Check sheet for the modelled part. Datum: model origin and axes. Units: mm. A direction names the side the tool comes from. Round coordinates to 2 decimals unless told otherwise and drop trailing zeros. Loops run counter-clockwise (first coordinate to the right, second up) from the corner with the lowest first, then second, coordinate; pieces in that order, holes last. Notation, with made-up numbers: (17.25, -13) -> (45.25, -13) arc R12 ccw to (45.25, 2) -> close; hole circle Ø7 at (-2.75, -35.5). An arc over 180 degrees is marked (long way). Return JSON: item names as keys, results as strings.
Autodesk Inventor part; units mm, degrees
ref_plane "YZ Plane" through (0, 0, 0) normal (1, 0, 0) x (0, 1, 0)
ref_plane "XZ Plane" through (0, 0, 0) normal (0, 1, 0) x (-1, 0, 0)
ref_plane "XY Plane" through (0, 0, 0) normal (0, 0, 1) x (1, 0, 0)
sketch "Sketch1" plane through (0, 0, 0) normal (1, 0, 0) x (0, 1, 0)
  line L0 (920.75, 0) -> (0, 0)
  line L1 (0, 0) -> (920.75, 0)
  line L2 (-297.6389, 409.8513) -> (2710.7909, 409.8513) construction
  line L3 (2710.7909, 409.8513) -> (2710.7909, -1716.9746) construction
  line L4 (2710.7909, -1716.9746) -> (-297.6389, -1716.9746) construction
  line L5 (-297.6389, -1716.9746) -> (-297.6389, 409.8513) construction
  line L6 (0, 0) -> (920.75, 0)
  line L7 (920.75, 0) -> (920.75, 100.33)
  line L8 (0, 100.33) -> (920.75, 100.33)
  line L9 (0, 0) -> (0, 100.33)
  line L10 (0, 100.33) -> (0, 120.65)
  line L11 (0, 120.65) -> (920.75, 120.65)
  line L12 (920.75, 120.65) -> (920.75, 100.33)
  line L13 (0, 120.65) -> (0, 196.85)
  line L14 (920.75, 196.85) -> (920.75, 120.65)
  line L15 (477.9962, 0) -> (477.9962, -13.97)
  line L16 (477.9962, -13.97) -> (434.8162, -13.97)
  line L17 (434.8162, -13.97) -> (434.8162, 0)
  line L18 (133.294, 0) -> (133.294, -13.97)
  line L19 (133.294, -13.97) -> (90.114, -13.97)
  line L20 (90.114, -13.97) -> (90.114, 0)
  line L21 (769.0257, 0) -> (769.0257, -13.97)
  line L22 (769.0257, -13.97) -> (812.2057, -13.97)
  line L23 (812.2057, -13.97) -> (812.2057, 0)
  line L24 (434.8162, -13.97) -> (477.9962, -13.97)
  line L25 (769.0257, -13.97) -> (812.2057, -13.97)
  line L26 (90.114, -13.97) -> (133.294, -13.97)
  line L27 (90.114, -13.97) -> (111.704, -13.97)
  line L28 (111.704, -13.97) -> (100.909, -13.97)
  line L29 (100.909, -13.97) -> (122.499, -13.97)
  line L30 (122.499, -13.97) -> (122.499, -33.02)
  line L31 (122.499, -33.02) -> (100.909, -33.02)
  line L32 (100.909, -33.02) -> (100.909, -13.97)
  line L33 (434.8162, -13.97) -> (456.4062, -13.97)
  line L34 (456.4062, -13.97) -> (445.6112, -13.97)
  line L35 (445.6112, -13.97) -> (467.2012, -13.97)
  line L36 (467.2012, -13.97) -> (467.2012, -33.02)
  line L37 (467.2012, -33.02) -> (445.6112, -33.02)
  line L38 (445.6112, -33.02) -> (445.6112, -13.97)
  line L39 (769.0257, -13.97) -> (790.6157, -13.97)
  line L40 (790.6157, -13.97) -> (779.8207, -13.97)
  line L41 (779.8207, -13.97) -> (801.4107, -13.97)
  line L42 (801.4107, -13.97) -> (801.4107, -33.02)
  line L43 (801.4107, -33.02) -> (779.8207, -33.02)
  line L44 (779.8207, -33.02) -> (779.8207, -13.97)
  line L45 (434.8162, 0) -> (413.2262, 0)
  line L46 (413.2262, 0) -> (413.2262, -11.43)
  line L47 (413.2262, -11.43) -> (371.9512, -11.43)
  line L48 (371.9512, -11.43) -> (371.9512, 64.77)
  arc A0 (413.2262, 72.0379) -> (371.9512, 72.0379) centre (392.5887, 68.404) ccw
  line L49 (413.2262, 0) -> (413.2262, 64.77)
  line L50 (371.9512, 64.77) -> (371.9512, 72.0379)
  line L51 (413.2262, 64.77) -> (413.2262, 72.0379)
  line L52 (434.8162, -13.97) -> (434.8162, 202.565)
  line L53 (477.9962, -13.97) -> (477.9962, 202.565)
  line L54 (769.0257, -13.97) -> (769.0257, 202.565)
  line L55 (812.2057, -13.97) -> (812.2057, 202.565)
  line L56 (812.2057, 202.565) -> (769.0257, 202.565)
  line L57 (477.9962, 202.565) -> (434.8162, 202.565)
  line L58 (133.294, -13.97) -> (133.294, 182.245)
  line L59 (90.114, -13.97) -> (90.114, 182.245)
  line L60 (90.114, 182.245) -> (133.294, 182.245)
  line L61 (67.3834, 182.245) -> (164.6776, 182.245)
  line L62 (413.2262, 202.565) -> (508.4774, 202.565)
  line L63 (745.5808, 202.565) -> (847.3717, 202.565)
  line L64 (67.3834, 161.925) -> (164.6776, 161.925)
  line L65 (413.2262, 182.245) -> (508.4774, 182.245)
  line L66 (745.5808, 182.245) -> (847.3717, 182.245)
  line L67 (133.294, -13.97) -> (133.294, 78.74)
  line L68 (133.294, 78.74) -> (434.8162, 78.74)
  line L69 (133.294, -13.97) -> (133.294, 26.67)
  line L70 (133.294, 26.67) -> (371.9512, 26.67)
  line L71 (133.294, 26.67) -> (298.394, 26.67)
  line L72 (298.394, 26.67) -> (317.7759, 78.74)
  line L73 (133.294, 78.74) -> (133.294, 59.055)
  line L74 (133.294, 59.055) -> (310.4486, 59.055)
  line L75 (371.9512, 0) -> (371.9512, -5.715)
  line L76 (371.9512, -5.715) -> (413.2262, -5.715)
  dimension "d0" = 920.75
  dimension "d1" = 20.32
  dimension "d2" = 76.2
  dimension "d3" = 13.97
  dimension "d4" = 43.18
  dimension "d5" = 13.97
  dimension "d6" = 43.18
  dimension "d7" = 13.97
  dimension "d8" = 13.97
  dimension "d9" = 43.18
  dimension "d10" = 21.59
  dimension "d11" = 19.05
  dimension "d12" = 21.59
  dimension "d13" = 19.05
  dimension "d14" = 21.59
  dimension "d15" = 19.05
  dimension "d16" = 21.59
  dimension "d17" = 11.43
  dimension "d18" = 41.275
  dimension "d19" = 76.2
  dimension "d20" = 20.955
  dimension "d21" = 216.535
  dimension "d22" = 216.535
  dimension "d23" = 216.535
  dimension "d24" = 216.535
  dimension "d25" = 196.215
  dimension "d26" = 20.32
  dimension "d27" = 20.32
  dimension "d28" = 20.32
  dimension "d29" = 92.71
  dimension "d30" = 40.64
  dimension "d31" = 165.1
  dimension "d32" = 19.685
extrude "Extrusion1" add sketch "Sketch1" along normal blind 5.715 and the other way blind 145.415 contours L46 L76 L48 L0 | L0 L48 L50 A0 L68 L51 L49 | L68 A0
sketch "Sketch2" plane through (-145.415, 413.2262, 72.0379) normal (0, 1, 0) x (1, 0, 0)
  line L0 (0, 0) -> (151.13, 0)
  line L1 (151.13, 77.7529) -> (151.13, 0)
  line L2 (0, 77.7529) -> (151.13, 77.7529)
  line L3 (0, 0) -> (0, 77.7529)
  line L4 (144.145, 70.7679) -> (144.145, 6.985)
  line L5 (144.145, 6.985) -> (6.985, 6.985)
  line L6 (6.985, 6.985) -> (6.985, 70.7679)
  line L7 (6.985, 70.7679) -> (144.145, 70.7679)
  line L8 (146.05, 72.6729) -> (146.05, 5.08)
  line L9 (146.05, 5.08) -> (5.08, 5.08)
  line L10 (5.08, 5.08) -> (5.08, 72.6729)
  line L11 (5.08, 72.6729) -> (146.05, 72.6729)
  line L12 (146.05, 5.08) -> (146.05, -20.9448)
  line L13 (146.05, 5.08) -> (172.0748, 5.08) construction
  line L14 (5.08, 5.08) -> (5.08, -29.2393)
  line L15 (5.08, -29.2393) -> (146.05, -20.9448)
  point P0 (145.415, 72.0379)
  dimension "d39" = 6.985
  dimension "d40" = 1.905
  dimension "d41" = 90
extrude "Extrusion2" cut sketch "Sketch2" against normal through all contours L14 L9 L12 L0 | L0 L12 L15 L14 | L10 L11 L8 L9 | L4 L5 L6 L7
sketch "Sketch3" plane through (5.715, 0, 0) normal (1, 0, 0) x (0, 0, -1)
  arc A0 (-72.0379, 413.2262) -> (-72.0379, 371.9512) centre (-68.404, 392.5887) ccw
  circle A1 centre (-68.404, 392.5887) radius 6.6675
  point P0 (0, 0)
  dimension "d44" = 13.335
sketch "Sketch4" plane through (-145.415, 0, 0) normal (-1, 0, 0) x (0, 0, 1)
  circle A0 centre (68.404, 392.5887) radius 6.6675
  circle A1 centre (68.404, 392.5887) radius 6.6675
  point P0 (0, 0)
extrude "Extrusion3" add sketch "Sketch4" along normal blind 3.175
extrude "Extrusion4" add sketch "Sketch3" along normal blind 3.175
fillet "Fillet1" radius 2.286 2 edges at (8.89, 392.5887, 75.0715) (-148.59, 392.5887, 61.7365)
sketch "Sketch5" plane through (5.715, 0, 0) normal (1, 0, 0) x (0, 0, -1)
  arc A0 (-72.0379, 413.2262) -> (-72.0379, 371.9512) centre (-68.404, 392.5887) ccw
  line L0 (-89.359, 392.5887) -> (-89.359, 351.6635)
  line L1 (5.715, 371.9512) -> (5.715, 413.2262)
  line L2 (-72.0379, 371.9512) -> (5.715, 371.9512)
  line L3 (5.715, 413.2262) -> (-72.0379, 413.2262)
  point P0 (0, 0)
  dimension "d50" = 95.0739
  dimension "d51" = 41.275
sketch "Sketch6" plane through (5.715, 413.2262, -5.715) normal (0, 0, -1) x (-1, 0, 0)
  line L0 (154.305, -16.256) -> (154.305, -25.019)
  line L1 (-3.175, -25.019) -> (-3.175, -16.256)
  point P0 (5.715, -413.2262)
  dimension "d52" = 157.48
properties part number "small side peice"
Q1. Material ranges on line 1 (X direction, y = 386.5, z = 52.5) (3 decimals); line 2 (Z direction, x = -139.5, y = 402) (3 decimals); line 3 (X direction, y = 392, z = -1) (3 decimals), recorded low to high.
Results list:
{"line 1": "-145.415 to -140.335, 0.635 to 5.715", "line 2": "-5.715 to -0.635", "line 3": "-145.415 to 5.715"}
Q2. Section check C-C (x = -58.5). Record the boundary of the cut face in (y, z) (3 decimals).
Results list:
{"outline": "(371.951, -5.715) -> (413.226, -5.715) -> (413.226, -0.635) -> (371.951, -0.635) -> close"}
Q3. Section check A-A (z = 51). Record the boundary of the cut face in (x, y) (3 decimals).
Results list:
{"outline": "(-145.415, 371.951) -> (-140.335, 371.951) -> (-140.335, 413.226) -> (-145.415, 413.226) -> close; (0.635, 371.951) -> (5.715, 371.951) -> (5.715, 413.226) -> (0.635, 413.226) -> close"}
Q4. Section check B-B (y = 380). Record the boundary of the cut face in (x, z) (3 decimals), then the cut area to 3 significant figures.
Results list:
{"outline": "(-145.415, -5.715) -> (5.715, -5.715) -> (5.715, 85.156) -> (0.635, 85.156) -> (0.635, -0.635) -> (-140.335, -0.635) -> (-140.335, 85.156) -> (-145.415, 85.156) -> close", "area": "1,640 mm^2"}
Q5. Tool access check on faces 5 (the cylindrical face through (6.153, 386.967, 64.82)), 6 (the cylindrical face through (-145.85, 386.97, 71.99)), 7 (the flat face through (-71, 393, -0.635)). Record the directions out of +Z, -Z, +X, -X, +Y, -Y that give a thin tool (end or side, any length) a straight path to the whole face; none if there is none.
Results list:
{"face 5": "+X", "face 6": "-X", "face 7": "+Z, +Y, -Y"}
Q6. Draft check along X on faces 1 (the flat face through (0.635, 393, 44)), 2 (the flat face through (-140.335, 393, 44)), 3 (the cylindrical face through (3.139, 392.179, 89.355)), 4 (the flat face through (-148.59, 393, 68)). Enter one of: released by +X, released by -X, zero draft, split by the parting line, or undercut.
Results list:
{"face 1": "undercut", "face 2": "undercut", "face 3": "zero draft", "face 4": "released by -X"}
Q7. Section check D-D (y = 401). Record the boundary of the cut face in (x, z) (3 decimals), then the cut area to 3 significant figures.
Results list:
{"outline": "(-145.415, -5.715) -> (5.715, -5.715) -> (5.715, 87.597) -> (0.635, 87.597) -> (0.635, -0.635) -> (-140.335, -0.635) -> (-140.335, 87.597) -> (-145.415, 87.597) -> close", "area": "1,660 mm^2"}
Q8. Go/stop test with flat-tipped pins: pin 1 (6 mm diameter, centred on y = 389, z = 5.5, fed in from -X) (3 decimals); pin 2 (20.5 mm diameter, centred on y = 384.5, z = 29.5, fed in from +X) (3 decimals). Record where each tip stops, or that it passes through.
Results list:
{"pin 1": "x = -145.415", "pin 2": "x = 5.715"}
